Work out the finished part from the listing and answer in its coordinate system (mm). Round coordinates to 2 decimals unless told otherwise and drop trailing zeros. Order: outer loops, then holes, each group sorted by start corner. A loop starts at its lowest first (then second) coordinate and runs counter-clockwise, first axis right, second up. Notation, with made-up numbers: (23.5, 26) -> (48.5, 26) arc R18 cw to (48.5, 41) -> close; hole circle Ø6 at (-38.75, 17.5). An arc over 180 degrees is marked (long way). Use one line per item in the form item = value.
```python
from build123d import *

# Parameters (mm, degrees)
BOSS_EXTRUDE1_DEPTH = 2
CHAMFER1_SIZE       = 1
FILLET1_R           = 5
SKETCH2_R           = 2.5
CUT_EXTRUDE1_DEPTH  = 3
SKETCH3_R           = 2.75
CUT_EXTRUDE2_DEPTH  = 3
CHAMFER2_SIZE2      = 2.383507185
CHAMFER2_SIZE       = 2
CHAMFER3_SIZE       = 1.7
CHAMFER3_SIZE_2     = 1.426469373


# Some blends are built 0.0001 mm under size
with BuildPart() as part:
    # Sketch1 → Boss-Extrude1 (new body)
    with BuildSketch(Plane(origin=(0, 0, 0), x_dir=(1, 0, 0), z_dir=(0, 1, 0))):
        Polygon((25, 5), (25, 13), (45, 13), (45, -13), (25, -13), (25, -5), (-25, -5), (-25, 5), align=None)
    extrude(amount=BOSS_EXTRUDE1_DEPTH)

    # Chamfer1
    chamfer1_edges = [part.edges().sort_by_distance(p)[0] for p in [
        (-25, 1, 5),
        (-25, 1, -5),
    ]]
    chamfer(chamfer1_edges, length=CHAMFER1_SIZE)

    # Fillet1
    fillet1_edges = [part.edges().sort_by_distance(p)[0] for p in [
        (25, 1, -13),
        (45, 1, -13),
        (45, 1, 13),
        (25, 1, 13),
    ]]
    fillet(fillet1_edges, radius=FILLET1_R)

    # Sketch2 → Cut-Extrude1 (cut)
    with BuildSketch(Plane(origin=(0, 2, 0), x_dir=(1, 0, 0), z_dir=(0, 1, 0))):
        with Locations(Location((40, 0, 0), (0, 0, 270))):
            Circle(SKETCH2_R)
    extrude(amount=-CUT_EXTRUDE1_DEPTH, mode=Mode.SUBTRACT)

    # Sketch3 → Cut-Extrude2 (cut)
    with BuildSketch(Plane(origin=(0, 2, 0), x_dir=(1, 0, 0), z_dir=(0, 1, 0))):
        with Locations(Location((13, 0, 0), (0, 0, 270))):
            Circle(SKETCH3_R)
        with Locations(Location((5, 0, 0), (0, 0, 270))):
            Circle(SKETCH3_R)
        with Locations(Location((-19, 0, 0), (0, 0, 270))):
            Circle(SKETCH3_R)
    extrude(amount=-CUT_EXTRUDE2_DEPTH, mode=Mode.SUBTRACT)

    # Chamfer2
    chamfer2_edges = [part.edges().sort_by_distance(p)[0] for p in [
        (-25, 2, 0),
    ]]
    chamfer2_side = [part.faces().sort_by_distance(p)[0] for p in [
        (-25, 1.96, 0),
    ]]
    chamfer(chamfer2_edges, length=CHAMFER2_SIZE - 0.0001, length2=CHAMFER2_SIZE2 - 0.0001, reference=chamfer2_side[0])  # a hair under: the kernel refuses the full size

    # Chamfer3
    # the kernel refuses this chamfer: 1.7, 1.426469373 mm, written as the material it takes off along each edge
    with BuildSketch(Plane(origin=(13, 2, 0), x_dir=(0, 0, 1), z_dir=(-1, 0, 0))) as chamfer3_piece_1:
        Polygon((2.75 + CHAMFER3_SIZE, 0), (2.75, -CHAMFER3_SIZE_2), (2.75, 0), align=None)
    revolve(axis=Axis((13, 2, 0), (0, 1, 0)), mode=Mode.SUBTRACT)
    with BuildSketch(Plane(origin=(5, 2, 0), x_dir=(0, 0, 1), z_dir=(-1, 0, 0))) as chamfer3_piece_2:
        Polygon((2.75 + CHAMFER3_SIZE, 0), (2.75, -CHAMFER3_SIZE_2), (2.75, 0), align=None)
    revolve(axis=Axis((5, 2, 0), (0, 1, 0)), mode=Mode.SUBTRACT)
    with BuildSketch(Plane(origin=(-19, 2, 0), x_dir=(0, 0, 1), z_dir=(-1, 0, 0))) as chamfer3_piece_3:
        Polygon((2.75 + CHAMFER3_SIZE, 0), (2.75, -CHAMFER3_SIZE_2), (2.75, 0), align=None)
    revolve(axis=Axis((-19, 2, 0), (0, 1, 0)), mode=Mode.SUBTRACT)


solid = part.part
```
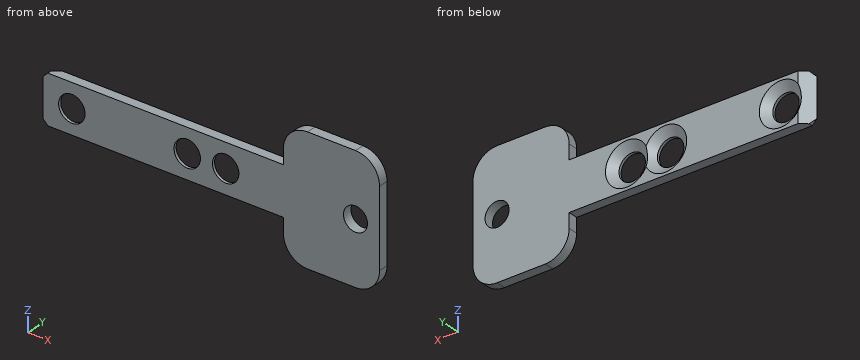
Item 1: The part is cut by section C-C, the plane y = 1.6. Give the vertices of the cut face in (x, z), and give its area (3 significant figures).
Findings:
outline = (-23.09, -5) -> (25, -5) -> (25, -8) arc R5 ccw to (30, -13) -> (40, -13) arc R5 ccw to (45, -8) -> (45, 8) arc R5 ccw to (40, 13) -> (30, 13) arc R5 ccw to (25, 8) -> (25, 5) -> (-23.09, 5) -> close; hole circle Ø7.95 at (-19, 0); hole circle Ø7.95 at (5, 0); hole circle Ø7.95 at (13, 0); hole circle Ø5 at (40, 0)
area = 811 mm^2
Item 2: Consider line 1 along X through (y, z) = (1.7, -0.25); line 2 along X through (y, z) = (0.1, 0); line 3 along X through (y, z) = (0.3, 0). Determine where each line is inside the solid, lowest interval first.
Findings:
line_1 = -14.92 to 0.92, 17.08 to 37.51, 42.49 to 45
line_2 = -24.88 to -21.75, -16.25 to 2.25, 7.75 to 10.25, 15.75 to 37.5, 42.5 to 45
line_3 = -24.64 to -21.75, -16.25 to 2.25, 7.75 to 10.25, 15.75 to 37.5, 42.5 to 45
Item 3: The part is cut by section B-B, the plane z = 0. Give the number of separate pieces and of enclosed holes in the cut face, and give its area (3 significant figures).
Findings:
separate_pieces = 5
enclosed_holes = 0
area = 87.7 mm^2
Item 4: The part is cut by section D-D, the plane z = 6.75. Give the vertices of the cut face in (x, y), and give its area (3 significant figures).
Findings:
outline = (25, 0) -> (45, 0) -> (45, 2) -> (25, 2) -> close
area = 40.0 mm^2
Item 5: The part is cut by section A-A, the plane x = 13. Give the vertices of the cut face in (y, z).
Findings:
outline = (0, -5) -> (2, -5) -> (2, -4.45) -> (0.57, -2.75) -> (0, -2.75) -> close; (0, 2.75) -> (0.57, 2.75) -> (2, 4.45) -> (2, 5) -> (0, 5) -> close
Item 6: Flat-ended cylindrical pins translate along their axes: P1, Ø9, axis at x = -19, z = 0, coming from the -Y side; P2, Ø0.6, axis at y = 1, z = 6.5, coming from the -X side; P3, Ø7, axis at x = 13, z = 0, coming from the +Y side. Find the tip coordinate at first contact, or state that the pin passes through.
Findings:
P1 = 0
P2 = 25
P3 = 1.2
